from build123d import *

# Parameters (mm, degrees)
F1_DEPTH = 1.5875
F3_DEPTH = 1.5875
F4_R     = 2.15265
F5_DEPTH = 1.5875


with BuildPart() as f1:
    # F0 (on Top) → F1 (new body)
    with BuildSketch(Plane.XY):
        Polygon((304.8, -344.8862546), (304.8, 0), (284.3822715367, 76.2), (228.6, 131.9822715367), (152.4, 152.4), (76.2, 131.9822715367), (20.4177284633, 76.2), (0, 0), (0, -344.8862546), (20.4177284633, -421.0862546), (76.2, -476.8685261367), (152.4, -497.2862546), (228.6, -476.8685261367), (284.3822715367, -421.0862546), align=None)
    extrude(amount=F1_DEPTH)

    # F2 (on face) → F3 (cut, through all)
    with BuildSketch(Plane.XY.offset(1.5875)):
        Polygon((278.5039850176, -344.8862546), (278.5039850176, 0), (261.6092545437, 63.0519925088), (215.4519925088, 109.2092545437), (152.4, 126.1039850176), (89.3480074912, 109.2092545437), (43.1907454563, 63.0519925088), (26.2960149824, 0), (26.2960149824, -344.8862546), (43.1907454563, -407.9382471088), (89.3480074912, -454.0955091437), (152.4, -470.9902396176), (215.4519925088, -454.0955091437), (261.6092545437, -407.9382471088), align=None)
    extrude(amount=-F3_DEPTH, mode=Mode.SUBTRACT)

    # F4 (on face) → F5 (join, through all)
    with BuildSketch(Plane.XY.offset(1.5875)):
        with BuildLine():
            Line((246.6607195716, 78.0005274808), (230.4005274808, 94.2607195716))
            Line((230.4005274808, 94.2607195716), (230.4005274808, 82.7630274808))
            ThreePointArc((230.4005274808, 82.7630274808), (231.7954314354, 79.3954314354), (235.1630274808, 78.0005274808))
            Line((235.1630274808, 78.0005274808), (246.6607195716, 78.0005274808))
        make_face()
        with Locations((235.1630274808, 82.7630274808)):
            Circle(F4_R, mode=Mode.SUBTRACT)
        with BuildLine():
            ThreePointArc((69.6369725192, 78.0005274808), (73.0045685646, 79.3954314354), (74.3994725192, 82.7630274808))
            Line((74.3994725192, 82.7630274808), (74.3994725192, 94.2607195716))
            Line((74.3994725192, 94.2607195716), (58.1392804284, 78.0005274808))
            Line((58.1392804284, 78.0005274808), (69.6369725192, 78.0005274808))
        make_face()
        with Locations((69.6369725192, 82.7630274808)):
            Circle(F4_R, mode=Mode.SUBTRACT)
        with BuildLine():
            Line((69.6369725192, -422.8867820808), (58.1392804284, -422.8867820808))
            Line((58.1392804284, -422.8867820808), (74.3994725192, -439.1469741716))
            Line((74.3994725192, -439.1469741716), (74.3994725192, -427.6492820808))
            ThreePointArc((74.3994725192, -427.6492820808), (73.0045685646, -424.2816860354), (69.6369725192, -422.8867820808))
        make_face()
        with Locations((69.6369725192, -427.6492820808)):
            Circle(F4_R, mode=Mode.SUBTRACT)
        with BuildLine():
            Line((230.4005274808, -439.1469741716), (246.6607195716, -422.8867820808))
            Line((246.6607195716, -422.8867820808), (235.1630274808, -422.8867820808))
            ThreePointArc((235.1630274808, -422.8867820808), (231.7954314354, -424.2816860354), (230.4005274808, -427.6492820808))
            Line((230.4005274808, -427.6492820808), (230.4005274808, -439.1469741716))
        make_face()
        with Locations((235.1630274808, -427.6492820808)):
            Circle(F4_R, mode=Mode.SUBTRACT)
    extrude(amount=-F5_DEPTH)


solid = f1.part
Geometry check sheet. Reference: the model listing, model coordinates, mm. A direction names the side the tool comes from. Round coordinates to 2 decimals unless told otherwise and drop trailing zeros. Write each loop counter-clockwise with the first axis right and the second up, starting at its lowest first coordinate (ties: lowest second). Pieces come first, ordered by that corner, then holes. Notation, with made-up numbers: (-38.5, 27) -> (-26.5, 27) arc R16 ccw to (-26.5, 40) -> close; hole circle Ø8 at (51.5, 33.5). An arc over 180 degrees is marked (long way). One line per item, written item: value. Start each with the question number.
(1) Draft check along X on faces 3 (the flat face through (120.433, -462.425, 0.805)), 4 (the flat face through (191.03, 142.05, 0.78)), 5 (the flat face through (48.7, 104.48, 0.78)). Enter one of: +X half, -X half, draft (parallel to the pull), parting line (faces both ways), or undercut.
(2) Scan lines: line 1 (X direction, y = -202.5, z = 1.35); line 2 (X direction, y = 105.5, z = 1.2); line 3 (Y direction, x = 244.5, z = 1.3). Record each from-to range of solid material in increasing order. Write a range as [from, to].
(3) Cross-section at C-C, the plane z = 0.5. Give the number of separate pieces and of enclosed holes in the cut face, and give its area (3 significant figures).
(4) Cross-section at A-A, the plane y = -109.5. Record the cut outline in (x, z).
(5) Go/stop test with flat-tipped pins: pin 1 Ø4 at (x, y) = (235.16, 82.76) entering from -Z; pin 2 Ø0.8 at (y, z) = (-432, 0.5) entering from -X; pin 3 Ø0.8 at (x, z) = (240, 1) entering from -Y; pin 4 Ø0.8 at (x, z) = (244, 1) entering from +Y. Record where each tip stops, or that it passes through.
(6) Cross-section at B-B, the plane x = 222. Record the cut outline in (y, z).
(7) Access from +Z, -Z, +X, -X, +Y, -Y to the whole of each face (thin tool, end or side, straight path). Record for faces 1 (the flat face through (254.03, -415.52, 0.8)), 2 (the flat face through (294.45, -383.52, 0.78)).
Answer:
1. face 3: undercut
1. face 4: +X half
1. face 5: -X half
2. line 1: [0, 26.3], [278.5, 304.8]
2. line 2: [49.72, 85.64], [219.16, 255.08]
2. line 3: [-460.97, -422.89], [78, 116.08]
3. separate pieces: 1
3. enclosed holes: 5
3. area: 40,600 mm²
4. outline: (0, 0) -> (26.3, 0) -> (26.3, 1.59) -> (0, 1.59) -> close; (278.5, 0) -> (304.8, 0) -> (304.8, 1.59) -> (278.5, 1.59) -> close
5. pin 1: through
5. pin 2: x = 30.93
5. pin 3: y = -465.87
5. pin 4: y = 116.98
6. outline: (-478.64, 0) -> (-447.55, 0) -> (-447.55, 1.59) -> (-478.64, 1.59) -> close; (102.66, 0) -> (133.75, 0) -> (133.75, 1.59) -> (102.66, 1.59) -> close
7. face 1: +Z, -Z
7. face 2: +Z, -Z, +X, -Y
